Verification items for the finished model (mm, model axes). A direction names the side the tool comes from. Round coordinates to 2 decimals unless told otherwise and drop trailing zeros. Order: outer loops, then holes, each group sorted by start corner. A loop starts at its lowest first (then second) coordinate and runs counter-clockwise, first axis right, second up. Notation, with made-up numbers: (14.25, 26.5) -> (21.25, 26.5) arc R17 cw to (21.25, 31.5) -> close; hole circle Ø3 at (79, 73.5). An arc over 180 degrees is marked (long way). Put each result on its own line as item: value.
```python
from build123d import *


with BuildPart() as part:
    # Sketch1 → Revolve1 (revolve)
    with BuildSketch(Plane.XZ):
        Polygon((6.5, 1.25), (6.25, 1.5), (5.25, 1.5), (5.25, 1), (3.75, 1), (3.75, 1.5), (3, 1.5), (3, -2.5), (3.75, -2.5), (3.75, -2), (5.25, -2), (5.25, -2.5), (6.25, -2.5), (6.5, -2.25), align=None)
    revolve(axis=Axis((1.5, 0, 2.5), (0, 0, -1)))


solid = part.part
```
Item 1: Sectioned sample at A-A, the plane x = 1.5. Record the boundary of the cut face in (y, z).
Geometry check:
outline: (-5, -2.25) -> (-4.75, -2.5) -> (-3.75, -2.5) -> (-3.75, -2) -> (-2.25, -2) -> (-2.25, -2.5) -> (-1.5, -2.5) -> (-1.5, 1.5) -> (-2.25, 1.5) -> (-2.25, 1) -> (-3.75, 1) -> (-3.75, 1.5) -> (-4.75, 1.5) -> (-5, 1.25) -> close; (1.5, -2.5) -> (2.25, -2.5) -> (2.25, -2) -> (3.75, -2) -> (3.75, -2.5) -> (4.75, -2.5) -> (5, -2.25) -> (5, 1.25) -> (4.75, 1.5) -> (3.75, 1.5) -> (3.75, 1) -> (2.25, 1) -> (2.25, 1.5) -> (1.5, 1.5) -> close
Item 2: Depth check by flat-ended pin: pin 1 Ø1 at (y, z) = (1.5, -2) entering from -X. Enter the tip coordinate at first touch or a pass-through.
Geometry check:
pin 1: x = -3.4
Item 3: Release check for a two-part mould opening along X. For faces 1 (the face through (3.646, -0.676, 1.254)), 2 (the face through (5, 2, 1.5)), 3 (the face through (3.646, -0.676, -2.246)), 4 (the face through (6.27, -1.5, -0.48)) record: pulls with the +X half, pulls with the -X half, needs draft (parallel to the pull), parting line crosses it, or undercut.
Geometry check:
face 1: undercut
face 2: needs draft
face 3: undercut
face 4: parting line crosses it
Item 4: Sectioned sample at C-C, the plane z = -0.1. Record the boundary of the cut face in (x, y), then the cut area to 3 significant figures.
Geometry check:
outline: circle Ø10 at (1.5, 0); hole circle Ø3 at (1.5, 0)
area: 71.5 mm2
Item 5: Sectioned sample at B-B, the plane y = 0. Record the boundary of the cut face in (x, z).
Geometry check:
outline: (-3.5, -2.25) -> (-3.25, -2.5) -> (-2.25, -2.5) -> (-2.25, -2) -> (-0.75, -2) -> (-0.75, -2.5) -> (0, -2.5) -> (0, 1.5) -> (-0.75, 1.5) -> (-0.75, 1) -> (-2.25, 1) -> (-2.25, 1.5) -> (-3.25, 1.5) -> (-3.5, 1.25) -> close; (3, -2.5) -> (3.75, -2.5) -> (3.75, -2) -> (5.25, -2) -> (5.25, -2.5) -> (6.25, -2.5) -> (6.5, -2.25) -> (6.5, 1.25) -> (6.25, 1.5) -> (5.25, 1.5) -> (5.25, 1) -> (3.75, 1) -> (3.75, 1.5) -> (3, 1.5) -> close
Item 6: Tool access check on faces 5 (the face through (0, 2, -2)), 6 (the face through (0.3, 0.9, -0.5)), 7 (the face through (3, 2, 1)). Record the directions out of +Z, -Z, +X, -X, +Y, -Y that give a thin tool (end or side, any length) a straight path to the whole face; none if there is none.
Geometry check:
face 5: -Z
face 6: +Z, -Z
face 7: +Z
Item 7: Material ranges on line 1 along X through (y, z) = (0, 1.2); line 2 along Y through (x, z) = (1.5, -2.2); line 3 along Y through (x, z) = (1.5, 0.1), recorded low to high.
Geometry check:
line 1: -3.5 to -2.25, -0.75 to 0, 3 to 3.75, 5.25 to 6.5
line 2: -5 to -3.75, -2.25 to -1.5, 1.5 to 2.25, 3.75 to 5
line 3: -5 to -1.5, 1.5 to 5
